from build123d import *

# Parameters (mm, degrees)
SKETCH2_W             = 24.295652174
SKETCH2_H             = 24.295652174
BOSS_EXTRUDE1_DEPTH   = 762
BOSS_EXTRUDE1_2_DEPTH = 762
SKETCH3_W             = 24.295652174
SKETCH3_H             = 25.4
BOSS_EXTRUDE2_DEPTH   = 558.8


with BuildPart() as part:
    # Sketch2 → Boss-Extrude1 (new body)
    with BuildSketch(Plane(origin=(0, 0, 0), x_dir=(1, 0, 0), z_dir=(0, 1, 0))):
        with Locations((12.147826087, 12.147826087)):
            Rectangle(SKETCH2_W, SKETCH2_H)
    extrude(amount=BOSS_EXTRUDE1_DEPTH)



with BuildPart() as body_2:
    # Sketch2 → Boss-Extrude1 2 (new body)
    with BuildSketch(Plane(origin=(0, 0, 0), x_dir=(1, 0, 0), z_dir=(0, 1, 0))):
        with Locations((12.147826087, 595.243478261)):
            Rectangle(SKETCH2_W, SKETCH2_H)
    extrude(amount=BOSS_EXTRUDE1_2_DEPTH)


with BuildPart() as part_1:
    add(part.part)

    add(body_2.part)  # Boss-Extrude2 merges body 2
    # Sketch3 → Boss-Extrude2 (add)
    with BuildSketch(Plane.XY.offset(-583.095652174)):
        with Locations((12.147826087, 749.3)):
            Rectangle(SKETCH3_W, SKETCH3_H)
    extrude(amount=BOSS_EXTRUDE2_DEPTH)


solid = part_1.part
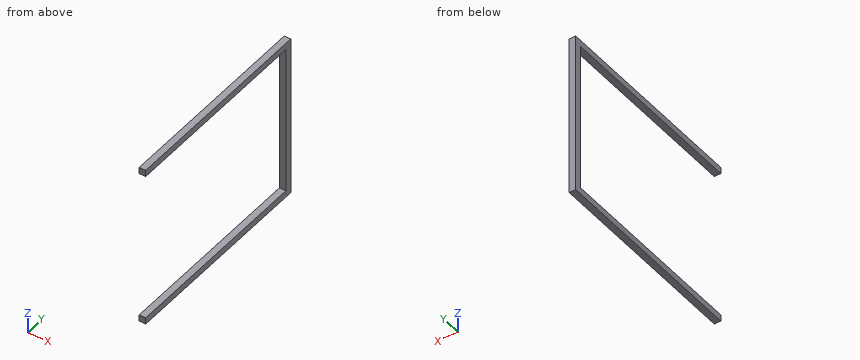
The listing builds one solid part. Answer for the finished solid, in the listing's coordinates (mm). Coordinates: 2 decimals unless noted, no trailing zeros. Loops run counter-clockwise (first coordinate to the right, second up) from the corner with the lowest first, then second, coordinate; pieces in that order, holes last. Notation, with made-up numbers: (47.5, 28) -> (75.5, 28) arc R26 cw to (75.5, 51) -> close; hole circle Ø9 at (62.25, -4.5). An arc over 180 degrees is marked (long way). Write item = value, one per line. Start each with the question number.
1) Given pin 1 Ø1 at (x, z) = (14.5, -479) entering from -Y, flat-ended and moving along its own axis, determine where the tip first touches the part or whether it passes through.
2) A cutting plane is placed at B-B (x = 7.5). Give the vertices of the cut face in (y, z), then the cut area to 3 significant figures.
3) A cutting plane is placed at A-A (y = 531). Give the vertices of the cut face in (x, z).
4) A cutting plane is placed at C-C (z = -235). Give the vertices of the cut face in (x, y), then the cut area to 3 significant figures.
5) Straight lines are drawn through the part: line 1 (Z direction, x = 3.5, y = 567); line 2 (Y direction, x = 5.5, z = -583). For each, find the intervals that lie inside material, in ascending order. Write a range as from..to.
Responses:
q1.pin_1 = 736.6
q2.outline = (0, -607.39) -> (762, -607.39) -> (762, 0) -> (0, 0) -> (0, -24.3) -> (736.6, -24.3) -> (736.6, -583.1) -> (0, -583.1) -> close
q2.area = 51,200 mm²
q3.outline = (0, -607.39) -> (24.3, -607.39) -> (24.3, -583.1) -> (0, -583.1) -> close; (0, -24.3) -> (24.3, -24.3) -> (24.3, 0) -> (0, 0) -> close
q4.outline = (0, 736.6) -> (24.3, 736.6) -> (24.3, 762) -> (0, 762) -> close
q4.area = 617 mm²
q5.line_1 = -607.39..-583.1, -24.3..0
q5.line_2 = 736.6..762
